Design review of the part built by this model. Coordinates are the model's own, in mm. Round coordinates to 2 decimals unless told otherwise and drop trailing zeros. Loops run counter-clockwise (first coordinate to the right, second up) from the corner with the lowest first, then second, coordinate; pieces in that order, holes last. Notation, with made-up numbers: (-23.75, 48.5) -> (30.25, 48.5) arc R19 ccw to (30.25, 61.5) -> close; hole circle Ø11 at (1.5, 85). An arc over 180 degrees is marked (long way). Answer as CSV lines item,"result". Start each with the question number.
(1) For P1, Ø4, axis at x = -11.5, y = 45.5, coming from the -Z side; P2, Ø2, axis at x = -53, z = 5.5, coming from the -Y side; P3, Ø2, axis at x = -42, z = 4, coming from the +Y side, all flat-tipped, find the tip position at first contact; note any pin that passes through.
(2) Take a section at A-A, the plane z = 5. Write out the cut boundary in (x, y).
(3) To check wall thickness, follow line 1 (Y direction, x = -46.5, z = 6.5); line 2 (X direction, y = 18, z = 3); line 3 (X direction, y = 21, z = 2). State the ranges of each line that lie inside material, in increasing order. Write a range as from..to.
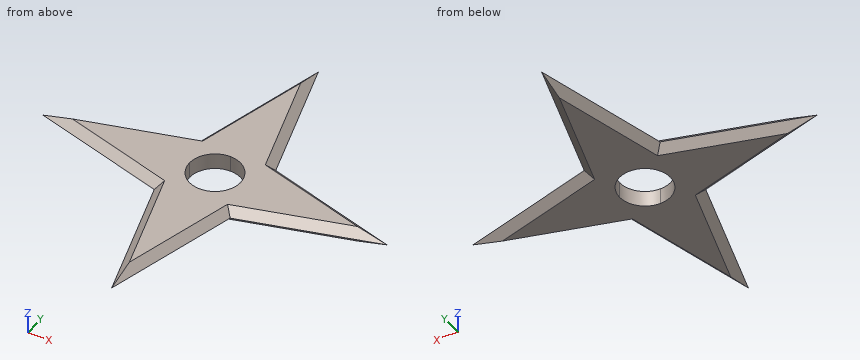
from build123d import *

# Parameters (mm, degrees)
F1_DEPTH = 7
F2_SIZE  = 3.5
F3_SIZE  = 3.49999


# Not quite as in the source:
# - a fillet or chamfer is up to 0.001 mm smaller than in the source, because OpenCascade refuses the exact size


with BuildPart() as f1:
    # F0 (on Top) → F1 (new body)
    with BuildSketch(Plane.XY):
        with BuildLine():
            ThreePointArc((-11.2, 0), (-7.9195959493, 7.9195959493), (0, 11.2))
            Line((0, 11.2), (0, 74.9999731779))
            Line((0, 74.9999731779), (-16.5413403588, 16.5413743234))
            Line((-16.5413403588, 16.5413743234), (-74.9999731779, 0))
            Line((-74.9999731779, 0), (-11.2, 0))
        make_face()
        with BuildLine():
            ThreePointArc((0, 11.2), (7.9195959493, 7.9195959493), (11.2, 0))
            Line((11.2, 0), (74.9999433756, 0))
            Line((74.9999433756, 0), (16.5414082881, 16.5413743234))
            Line((16.5414082881, 16.5413743234), (0, 74.9999731779))
            Line((0, 74.9999731779), (0, 11.2))
        make_face()
        with BuildLine():
            Line((74.9999433756, 0), (11.2, 0))
            ThreePointArc((11.2, 0), (7.9195959493, -7.9195959493), (0, -11.2))
            Line((0, -11.2), (0, -74.9999433756))
            Line((0, -74.9999433756), (16.5412724298, -16.5413063943))
            Line((16.5412724298, -16.5413063943), (74.9999433756, 0))
        make_face()
        with BuildLine():
            Line((0, -74.9999433756), (0, -11.2))
            ThreePointArc((0, -11.2), (-7.9195959493, -7.9195959493), (-11.2, 0))
            Line((-11.2, 0), (-74.9999731779, 0))
            Line((-74.9999731779, 0), (-16.5413403588, -16.5413063943))
            Line((-16.5413403588, -16.5413063943), (0, -74.9999433756))
        make_face()
    extrude(amount=F1_DEPTH)

    # F2
    f2_edges = [f1.edges().sort_by_distance(p)[0] for p in [
        (-45.770657, -8.270653, 7),
        (-8.27067, -45.770625, 7),
        (8.270636, -45.770625, 7),
        (45.770608, -8.270653, 7),
        (45.770676, 8.270687, 7),
        (8.270704, 45.770674, 7),
        (-8.27067, 45.770674, 7),
        (-45.770657, 8.270687, 7),
    ]]
    chamfer(f2_edges, length=F2_SIZE)

    # F3 (size 3.5 in the source; OpenCascade refuses exactly that, so slightly less here)
    f3_edges = [f1.edges().sort_by_distance(p)[0] for p in [
        (-45.770657, -8.270653, 0),
        (-45.770657, 8.270687, 0),
        (-8.27067, 45.770674, 0),
        (8.270704, 45.770674, 0),
        (45.770676, 8.270687, 0),
        (45.770608, -8.270653, 0),
        (8.270636, -45.770625, 0),
        (-8.27067, -45.770625, 0),
    ]]
    chamfer(f3_edges, length=F3_SIZE)


solid = f1.part
The answers:
1,P1,"through"
1,P2,"y = -5.22"
1,P3,"y = 9.58"
2,outline,"(-69.49, 0) -> (-15.33, -15.33) -> (0, -69.49) -> (15.33, -15.33) -> (69.49, 0) -> (15.33, 15.33) -> (0, 69.49) -> (-15.33, 15.33) -> close; hole circle Ø22.4 at (0, 0)"
3,line 1,"-4.95..4.95"
3,line 2,"-15.61..15.61"
3,line 3,"-13.72..13.72"
